The figure shows three views and two pictorial views of one solid part (mm, origin at its lowest corner). Answer the questions. A direction names the side the tool comes from. Coordinates: 2 decimals unless noted, no trailing zeros. Write each loop counter-clockwise with the first axis right and the second up, starting at its lowest first coordinate (ties: lowest second). Pieces come first, ordered by that corner, then holes.
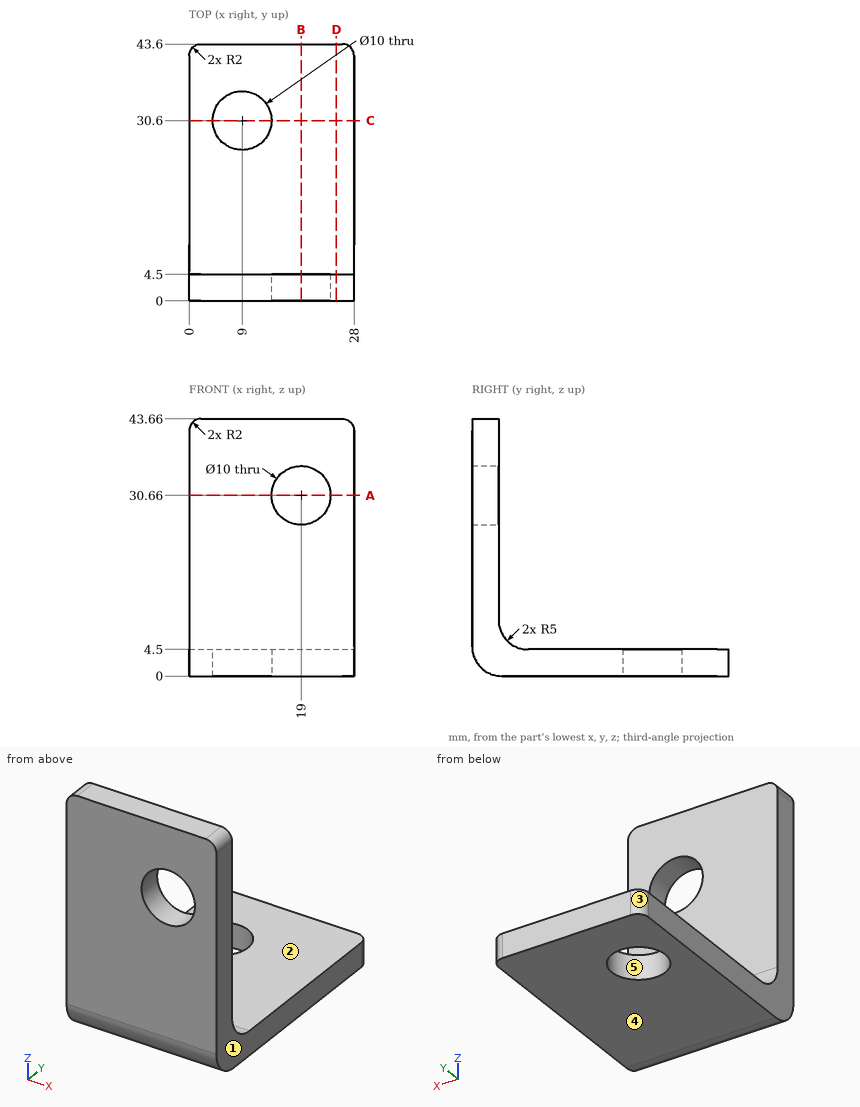
Item 1: The part is cut by section C-C (y = 30.6). Give the vertices of the cut face in (x, z), and give its area (3 significant figures).
Item 2: Find the intervals of material crossed by probe 1 along Z at (x, y) = (23.5, 11); probe 2 along Z at (x, y) = (19, 2.1); probe 3 along X at (y, z) = (30, 3), in increasing order.
Item 3: The part is cut by section A-A (z = 30.66). Give the vertices of the cut face in (x, y).
Item 4: The part is cut by section D-D (x = 25). Give the vertices of the cut face in (y, z).
Item 5: Determine the mould class of the marked faces 3, 4 and 5 for opening direction X: +X half, -X half, draft (parallel to the pull), parting line (faces both ways), or undercut.
Item 6: For the marked faces 1 and 2, determine the directions among +Z, -Z, +X, -X, +Y, -Y from which every point of the face is accessible in a straight line to the end or side of a thin tool.
Item 7: Given pin 1 (8 mm diameter, centred on x = 19, z = 30.66, fed in from +Y); pin 2 (14 mm diameter, centred on x = 13, y = 22, fed in from +Z), each flat-ended and moving along its own axis, determine where each tip first touches the part or whether it passes through.
Item 8: The part is cut by section B-B (x = 19). Give the vertices of the cut face in (y, z), and give its area (3 significant figures).
Answer:
1. outline: (0, 0) - (4, 0) - (4, 4.5) - (0, 4.5) - close; (14, 0) - (28, 0) - (28, 4.5) - (14, 4.5) - close
1. area: 81.0 mm2
2. probe 1: z = 0 to 4.5
2. probe 2: z = 0.93 to 25.66, 35.66 to 43.66
2. probe 3: x = 0 to 4.04, 13.96 to 28
3. outline: (0, 0) - (14, 0) - (14, 4.5) - (0, 4.5) - close; (24, 0) - (28, 0) - (28, 4.5) - (24, 4.5) - close
4. outline: (0, 5) arc R5 ccw to (5, 0) - (43.6, 0) - (43.6, 4.5) - (9.5, 4.5) arc R5 cw to (4.5, 9.5) - (4.5, 43.66) - (0, 43.66) - close
5. face 3: -X half
5. face 4: draft
5. face 5: undercut
6. face 1: +Z, -Z, +X, +Y, -Y
6. face 2: +Z, +X, -X, +Y
7. pin 1: passes through
7. pin 2: stops at z = 4.5
8. outline: (0, 5) arc R5 ccw to (5, 0) - (43.6, 0) - (43.6, 4.5) - (9.5, 4.5) arc R5 cw to (4.5, 9.5) - (4.5, 25.66) - (0, 25.66) - close; (0, 35.66) - (4.5, 35.66) - (4.5, 43.66) - (0, 43.66) - close
8. area: 327 mm2
